Autodesk Inventor part; units mm, degrees
ref_plane "YZ Plane" through (0, 0, 0) normal (1, 0, 0) x (0, 1, 0)
ref_plane "XZ Plane" through (0, 0, 0) normal (0, 1, 0) x (-1, 0, 0)
ref_plane "XY Plane" through (0, 0, 0) normal (0, 0, 1) x (1, 0, 0)
sketch "Sketch1" plane through (0, 0, 0) normal (0, 0, 1) x (1, 0, 0)
  line L0 (0, 0) -> (19.5, 0)
  line L1 (19.5, 0) -> (19.5, 19.5)
  line L2 (19.5, 19.5) -> (0, 19.5)
  line L3 (0, 19.5) -> (0, 0)
  dimension "d0" = 19.5
  dimension "d1" = 19.5
extrude "Extrusion1" add sketch "Sketch1" along normal blind 7.5
sketch "Sketch6" plane through (0, 0, 7.5) normal (0, 0, 1) x (1, 0, 0)
  line L0 (19.5, 0) -> (19.5, 19.5) construction
  line L1 (19.5, 9.75) -> (0, 9.75) construction
  line L2 (0, 19.5) -> (0, 0) construction
  circle A0 centre (9.75, 9.75) radius 6
  dimension "d14" = 12
sketch "Sketch7" plane through (0, 0, 0) normal (-1, 0, 0) x (0, 0, 1)
  line L0 (0, 19.5) -> (0, 0)
  line L1 (0, 0) -> (7.5, 0)
  line L2 (7.5, 19.5) -> (7.5, 0)
  line L3 (0, 19.5) -> (7.5, 19.5)
  dimension "d15" = 7.5
extrude "Extrusion4" add sketch "Sketch6" along normal blind 18
sketch "Sketch8" plane through (0, 19.5, 0) normal (0, 1, 0) x (1, 0, 0)
  line L0 (19.5, 0) -> (0, 0)
  line L1 (0, 0) -> (19.5, 0) construction
  line L2 (9.75, 0) -> (9.75, -5) construction
  line L3 (9.75, -5) -> (11.9374, -5) construction
  circle A0 centre (9.75, -4) radius 1
  dimension "d18" = 5
  dimension "d19" = 2
extrude "Extrusion5" cut sketch "Sketch8" against normal up to surface (19.5 mm away)
properties part number "HDzero runcam with micro spacer"
Model file for the job. Use its own axes, mm. A direction names the side the tool comes from. Round coordinates to 2 decimals unless told otherwise and drop trailing zeros. Order: outer loops, then holes, each group sorted by start corner. A loop starts at its lowest first (then second) coordinate and runs counter-clockwise, first axis right, second up. Notation, with made-up numbers: (42, 40) -> (65, 40) arc R9 cw to (65, 56) -> close; hole circle Ø6 at (-3, -22). An arc over 180 degrees is marked (long way). Use one line per item in the form item = value.
Item 1: Flat gauge pins, fed straight in: pin 1 Ø6 at (y, z) = (14, 15.5) entering from +X; pin 2 Ø4 at (x, y) = (15.5, 15.5) entering from +Z; pin 3 Ø2 at (x, z) = (4, 13.5) entering from +Y. Where does each tip first touch, or does it go through?
Returned:
pin_1 = 15.62
pin_2 = 7.5
pin_3 = 13.42
Item 2: Tool access for faces 4 (the face through (5, 14, 7.5)), 5 (the face through (10, 0, 2)): list every direction of +Z, -Z, +X, -X, +Y, -Y with a clear straight run to the whole face (end or side of a thin tool).
Returned:
face_4 = +Z
face_5 = +Z, -Z, +X, -X, -Y
Item 3: Cut at A-A, the plane x = 9.75. Write the cut outline in (y, z).
Returned:
outline = (0, 0) -> (19.5, 0) -> (19.5, 3) -> (0, 3) -> close; (0, 5) -> (19.5, 5) -> (19.5, 7.5) -> (15.75, 7.5) -> (15.75, 25.5) -> (3.75, 25.5) -> (3.75, 7.5) -> (0, 7.5) -> close
Item 4: Cut at D-D, the plane z = 12.25. Write the cut outline in (x, y).
Returned:
outline = circle Ø12 at (9.75, 9.75)
Item 5: Drill centre lines: line 1 (X direction, y = 5, z = 4); line 2 (Z direction, x = 9.75, y = 9); line 3 (Z direction, x = 15.5, y = 7.5). Where is each one in solid material? Low to high.
Returned:
line_1 = 0 to 8.75, 10.75 to 19.5
line_2 = 0 to 3, 5 to 25.5
line_3 = 0 to 7.5
Item 6: Pull direction Z, two halves, no side cores. Call faces 1 (the face through (9.013, 9.886, 3.324)), 2 (the face through (19.5, 10, 4)), 3 (the face through (10, 10, 0)): released by +Z, released by -Z, zero draft, split by the parting line, or undercut.
Returned:
face_1 = undercut
face_2 = zero draft
face_3 = released by -Z
Item 7: Cut at B-B, the plane z = 4. Write the cut outline in (x, y), and give its area (3 significant figures).
Returned:
outline = (0, 0) -> (8.75, 0) -> (8.75, 19.5) -> (0, 19.5) -> close; (10.75, 0) -> (19.5, 0) -> (19.5, 19.5) -> (10.75, 19.5) -> close
area = 341 mm^2
Item 8: Cut at C-C, the plane y = 9.75. Write the cut outline in (x, z).
Returned:
outline = (0, 0) -> (19.5, 0) -> (19.5, 7.5) -> (15.75, 7.5) -> (15.75, 25.5) -> (3.75, 25.5) -> (3.75, 7.5) -> (0, 7.5) -> close; hole circle Ø2 at (9.75, 4)
